```python
from build123d import *

# Parameters (mm, degrees)
BOSS_EXTRUDE1_DEPTH = 5
BOSS_EXTRUDE2_DEPTH = 9
SKETCH4_R           = 2.25
CUT_EXTRUDE1_DEPTH  = 6
SKETCH5_R           = 1.85
CUT_EXTRUDE2_DEPTH  = 5
SKETCH6_R           = 2
CUT_EXTRUDE3_DEPTH  = 5
SKETCH7_R           = 1.85
CUT_EXTRUDE4_DEPTH  = 5


with BuildPart() as part:
    # Sketch1 → Boss-Extrude1 (new body)
    with BuildSketch(Plane(origin=(0, 0, 0), x_dir=(1, 0, 0), z_dir=(0, 1, 0))):
        Polygon((-30, -8.5), (-12.413030788, -8.5), (-8.660254038, -15), (8.660254038, -15), (12.413030788, -8.5), (30, -8.5), (30, 8.5), (12.413030788, 8.5), (8.660254038, 15), (-8.660254038, 15), (-12.413030788, 8.5), (-30, 8.5), align=None)
        Polygon((-5.773502692, -10), (-11.547005384, 0), (-5.773502692, 10), (5.773502692, 10), (11.547005384, 0), (5.773502692, -10), align=None, mode=Mode.SUBTRACT)
    extrude(amount=BOSS_EXTRUDE1_DEPTH)

    # Sketch3 → Boss-Extrude2 (add)
    with BuildSketch(Plane(origin=(0, 5, 0), x_dir=(1, 0, 0), z_dir=(0, 1, 0))):
        Polygon((-14.43375673, 0), (-7.216878365, -12.5), (7.216878365, -12.5), (14.43375673, 0), (7.216878365, 12.5), (-7.216878365, 12.5), align=None)
        Polygon((-11.547005384, 0), (-5.773502692, -10), (5.773502692, -10), (11.547005384, 0), (5.773502692, 10), (-5.773502692, 10), align=None, mode=Mode.SUBTRACT)
    extrude(amount=BOSS_EXTRUDE2_DEPTH)

    # Sketch4 → Cut-Extrude1 (cut, through all)
    with BuildSketch(Plane(origin=(0, 5, 0), x_dir=(1, 0, 0), z_dir=(0, 1, 0))):
        with Locations(Location((-24, 0, 0), (0, 0, 270))):  # turned: the seam where the file's is
            Circle(SKETCH4_R)
    cut_extrude1 = extrude(amount=-CUT_EXTRUDE1_DEPTH, mode=Mode.SUBTRACT)

    # Mirror1: Cut-Extrude1 across plane
    add(cut_extrude1.mirror(Plane(origin=(0, 0, 0), x_dir=(0, 0, 1), z_dir=(1, 0, 0))), mode=Mode.SUBTRACT)

    # Sketch5 → Cut-Extrude2 (cut)
    with BuildSketch(Plane.XY.offset(15)):
        with Locations(Location((0, 9, 0), (0, 0, 180))):  # turned: the seam where the file's is
            Circle(SKETCH5_R)
    extrude(amount=-CUT_EXTRUDE2_DEPTH, mode=Mode.SUBTRACT)

    # Sketch6 → Cut-Extrude3 (cut)
    with BuildSketch(Plane(origin=(12.990381057, 0, -7.5), x_dir=(-0.5, 0, -0.866025404), z_dir=(0.866025404, 0, -0.5))):
        with Locations(Location((0, 9, 0), (0, 0, 180))):  # turned: the seam where the file's is
            Circle(SKETCH6_R)
    extrude(amount=-CUT_EXTRUDE3_DEPTH, mode=Mode.SUBTRACT)

    # Sketch7 → Cut-Extrude4 (cut)
    with BuildSketch(Plane(origin=(-12.990381057, 0, -7.5), x_dir=(-0.5, 0, 0.866025404), z_dir=(-0.866025404, 0, -0.5))):
        with Locations(Location((0, 9, 0), (0, 0, 180))):  # turned: the seam where the file's is
            Circle(SKETCH7_R)
    extrude(amount=-CUT_EXTRUDE4_DEPTH, mode=Mode.SUBTRACT)


solid = part.part
```
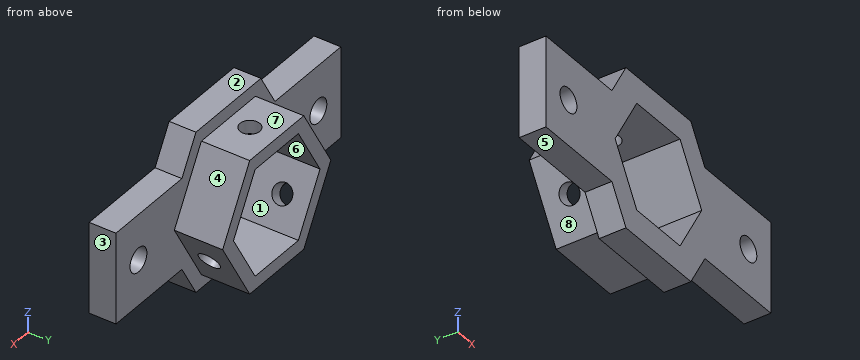
Here's how the part is built. I have some questions about the finished solid (model axes, mm). Face numbers are marked on the shaded views. A direction names the side the tool comes from. Round coordinates to 2 decimals unless told otherwise and drop trailing zeros. Write each loop counter-clockwise with the first axis right and the second up, starting at its lowest first coordinate (ties: lowest second). Pieces come first, ordered by that corner, then holes.
Q1. Please list where these lines run through material, in increasing order: probe 1 along X at (y, z) = (3.2, 0); probe 2 along Z at (x, y) = (-4.5, 4); probe 3 along Y at (x, z) = (0, 11.1).
Q2. If we section it at D-D on x = 0: Write out the boundary of the cut face in (y, z), plus the area to 4 significant figures.
Q3. Which directions (+Z, -Z, +X, -X, +Y, -Y) give clear straight access to the entire face, cutting with the end or side of a thin tool? Please do the marked faces 4, 5, 6, 7 and 8.
Q4. If we section it at C-C on y = 1.75: Write out the boundary of the cut face in (x, z), plus the area to 3 significant figures.
Q5. If we section it at A-A on x = -24: Write out the boundary of the cut face in (y, z).
Q6. If we section it at B-B on y = 12.75: Write out the boundary of the cut face in (x, z), plus the area to 3 significant figures.
Q7. If we mould it in two halves opening along Z, with no side actions, what happens to the marked faces 1, 2 and 3? For each: +Z half, -Z half, draft (parallel to the pull), parting line (faces both ways), or undercut.
Q8. Will these pins go through, and if not, where does the flat tip stop? P1, Ø4, axis at x = -20.5, z = 6, coming from the +Y side; P2, Ø4, axis at x = 23, y = 1.5, coming from the -Z side; P3, Ø6, axis at x = -1, y = 9.5, coming from the -Z side.
Answer below:
1. probe 1: x = -30 to -26.25, -21.75 to -11.55, 11.55 to 21.75, 26.25 to 30
1. probe 2: z = -15 to -10, 10 to 15
1. probe 3: y = 0 to 7.15, 10.85 to 14
2. outline: (0, -15) - (5, -15) - (5, -12.5) - (14, -12.5) - (14, -10) - (0, -10) - close; (0, 10) - (7.15, 10) - (7.15, 12.5) - (5, 12.5) - (5, 15) - (0, 15) - close; (10.85, 10) - (14, 10) - (14, 12.5) - (10.85, 12.5) - close
2. area: 85.75 mm2
3. face 4: +Z, +X, +Y
3. face 5: -Z, -X, +Y, -Y
3. face 6: +Y, -Y
3. face 7: +Z, +X, -X, +Y
3. face 8: -Z, -X, +Y
4. outline: (-30, -8.5) - (-12.41, -8.5) - (-8.66, -15) - (8.66, -15) - (12.41, -8.5) - (30, -8.5) - (30, 8.5) - (12.41, 8.5) - (8.66, 15) - (-8.66, 15) - (-12.41, 8.5) - (-30, 8.5) - close; hole circle Ø4.5 at (-24, 0); hole (-11.55, 0) - (-5.77, -10) - (5.77, -10) - (11.55, 0) - (5.77, 10) - (-5.77, 10) - close; hole circle Ø4.5 at (24, 0)
4. area: 916 mm2
5. outline: (0, -8.5) - (5, -8.5) - (5, -2.25) - (0, -2.25) - close; (0, 2.25) - (5, 2.25) - (5, 8.5) - (0, 8.5) - close
6. outline: (-14.43, 0) - (-7.22, -12.5) - (7.22, -12.5) - (14.43, 0) - (7.22, 12.5) - (-7.22, 12.5) - close; hole (-11.55, 0) - (-5.77, -10) - (5.77, -10) - (11.55, 0) - (5.77, 10) - (-5.77, 10) - close
6. area: 195 mm2
7. face 1: undercut
7. face 2: +Z half
7. face 3: draft
8. P1: stops at y = 5
8. P2: stops at z = -8.5
8. P3: stops at z = -12.5
